from build123d import *

# Parameters (mm, degrees)
SKETCH1_RX          = 82.55
SKETCH1_RY          = 53.975
SKETCH1_R           = 7.874
BOSS_EXTRUDE1_DEPTH = 12.7


with BuildPart() as part:
    # Sketch1 → Boss-Extrude1 (new body)
    with BuildSketch(Plane.XY):
        with Locations((0, 0)):
            Ellipse(SKETCH1_RX, SKETCH1_RY)
        with Locations((63.5, 0)):
            Circle(SKETCH1_R, mode=Mode.SUBTRACT)
        Polygon((-16.102954744, 0), (-27.101477372, 19.05), (-49.098522628, 19.05), (-60.097045256, 0), (-49.098522628, -19.05), (-27.101477372, -19.05), align=None, mode=Mode.SUBTRACT)
        with BuildLine():
            ThreePointArc((50.282192855, 13.718311641), (44.45, 0), (50.282192855, -13.718311641))
            ThreePointArc((50.282192855, -13.718311641), (52.194156422, -18.928772289), (49.279540311, -23.652067514))
            ThreePointArc((49.279540311, -23.652067514), (27.015068096, -33.914821935), (2.830078432, -37.92943602))
            ThreePointArc((2.830078432, -37.92943602), (-8.566993644, -31.572176432), (-8.342514151, -18.523896457))
            ThreePointArc((-8.342514151, -18.523896457), (-3.048, 0), (-8.342514151, 18.523896457))
            ThreePointArc((-8.342514151, 18.523896457), (-8.566993644, 31.572176432), (2.830078432, 37.92943602))
            ThreePointArc((2.830078432, 37.92943602), (27.015068096, 33.914821935), (49.279540311, 23.652067514))
            ThreePointArc((49.279540311, 23.652067514), (52.194156422, 18.928772289), (50.282192855, 13.718311641))
        make_face(mode=Mode.SUBTRACT)
    extrude(amount=BOSS_EXTRUDE1_DEPTH)


solid = part.part
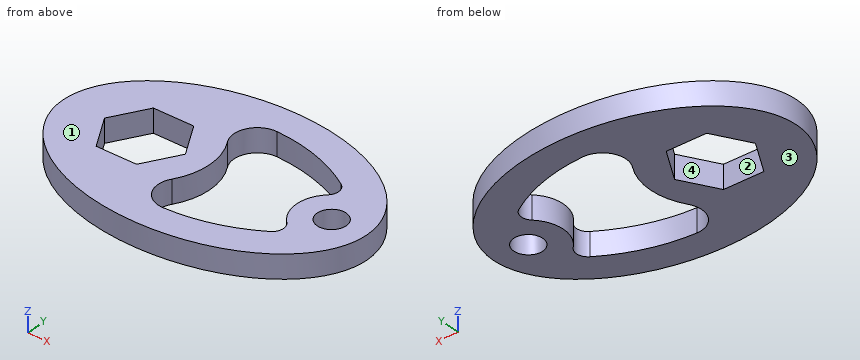
Source: CAD feature listing. Evaluate the final solid. Frame: model axes, mm. Face numbers are marked on the shaded views. A direction names the side the tool comes from. Coordinates: 2 decimals unless noted, no trailing zeros. Answer in a Markdown table with one row per item. Add a question column.
Q1. Ray query, line 1 along X through (y, z) = (5, 8); line 2 along Y through (x, z) = (63.5, 5.5); line 3 along Y through (x, z) = (59, 7.75). Return the intervals inside material, ascending.
Q2. Contact query for flat-ended pins moving along their axis: pin 1 Ø3 at (x, z) = (-53.5, 7) entering from -Y; pin 2 Ø4 at (x, z) = (-41, 5) entering from -Y; pin 3 Ø3 at (y, z) = (-3, 7.5) entering from -X. Output: stop coordinate, or through.
Q3. Pull-direction query (Y, two-part tool) for the marked faces 3 and 4; classes: pulls with the +Y half, pulls with the -Y half, needs draft (parallel to the pull), parting line crosses it, or undercut.
Q4. Section A-A on z = 3.5. Give the number of separate pieces and of enclosed holes in the cut face, and give its area (3 significant figures).
Q5. Reachability of the marked faces 1 and 2 from +Z, -Z, +X, -X, +Y, -Y: full face, straight path, thin tool, end or side. Return the list, or none.
Computed values:
| question | item | result |
|---|---|---|
| 1 | line 1 | x = -82.2 to -57.21, -18.99 to -3.41, 45.12 to 57.42, 69.58 to 82.2 |
| 1 | line 2 | y = -34.49 to -7.87, 7.87 to 34.49 |
| 1 | line 3 | y = -37.75 to -6.46, 6.46 to 37.75 |
| 2 | pin 1 | stops at y = -41.92 |
| 2 | pin 2 | stops at y = -47.57 |
| 2 | pin 3 | stops at x = -82.52 |
| 3 | face 3 | needs draft |
| 3 | face 4 | undercut |
| 4 | separate pieces | 1 |
| 4 | enclosed holes | 3 |
| 4 | area | 8,800 mm^2 |
| 5 | face 1 | +Z, +X, -X, +Y, -Y |
| 5 | face 2 | +Z, -Z |
